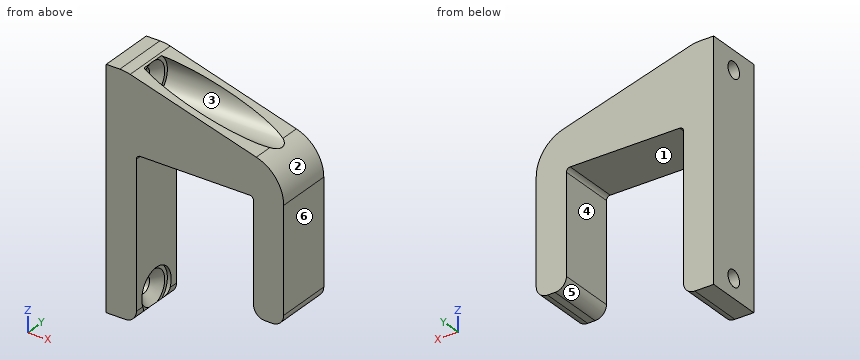
from build123d import *

# Parameters (mm, degrees)
BOSS_EXTRU_1_DEPTH                           = 7.5
CONG_1_R                                     = 1
CONG_2_R                                     = 10
CONG_3_R                                     = 3
CHAMBRAGE_POUR_VIS_T_TE_CYLINDRIQUE_AT_COUNT = 2
CHAMBRAGE_POUR_VIS_T_TE_CYLINDRIQUE_AT_PITCH = 52


with BuildPart() as part:
    # Esquisse1 → Boss.-Extru.1 (new, symmetric)
    with BuildSketch(Plane(origin=(0, 0, 0), x_dir=(1, 0, 0), z_dir=(0, 1, 0))):
        Polygon((0, 0), (0, 42), (-8, 42), (-8, -20), (-3, -20), (39, -8), (39, 30), (31, 30), (31, 0), align=None)
    extrude(amount=BOSS_EXTRU_1_DEPTH, both=True)

    # Congé1
    cong_1_edges = [part.edges().sort_by_distance(p)[0] for p in [
        (31, 0, 0),
        (0, 0, 0),
    ]]
    fillet(cong_1_edges, radius=CONG_1_R)

    # Congé2
    cong_2_edges = [part.edges().sort_by_distance(p)[0] for p in [
        (39, 0, 8),
        (-3, 0, 20),
    ]]
    fillet(cong_2_edges, radius=CONG_2_R)

    # Congé3
    cong_3_edges = [part.edges().sort_by_distance(p)[0] for p in [
        (31, 0, -30),
        (39, 0, -30),
        (0, 0, -42),
    ]]
    fillet(cong_3_edges, radius=CONG_3_R)

    # Esquisse2 → Chambrage pour vis à tête cylindrique à 6 pans creux (ou vis CHC) M41 (revolve, cut)
    with BuildSketch(Plane(origin=(0, 0, -37), x_dir=(0, 0, -1), z_dir=(0, 1, 0))):
        Polygon((0, 0), (0, 8), (2.15, 8), (2.15, 3.35), (4.5, 1), (5.5, 1), (5.5, 0), (5.5, -39), (0, -39), align=None)
    chambrage_pour_vis_t_te_cylindrique = revolve(axis=Axis((6.35, 0, -37), (-1, 0, 0)), mode=Mode.SUBTRACT)

    # Chambrage pour vis à tête cylindrique à 6 pans creux (ou vis CHC) M41 at: Chambrage pour vis à tête cylindrique à 6 pans creux (ou vis CHC) M41 ×2
    with Locations(*[(0, 0, i * CHAMBRAGE_POUR_VIS_T_TE_CYLINDRIQUE_AT_PITCH) for i in range(1, CHAMBRAGE_POUR_VIS_T_TE_CYLINDRIQUE_AT_COUNT)]):
        add(chambrage_pour_vis_t_te_cylindrique, mode=Mode.SUBTRACT)


solid = part.part
Design review of the part built by this model. Coordinates are the model's own, in mm. Face numbers are marked on the shaded views. A direction names the side the tool comes from. Coordinates: 2 decimals unless noted, no trailing zeros. Write each loop counter-clockwise with the first axis right and the second up, starting at its lowest first coordinate (ties: lowest second). Pieces come first, ordered by that corner, then holes. Notation, with made-up numbers: (-18.5, 81.25) - (-7.5, 81.25) arc R23 cw to (-7.5, 104.25) - close; hole circle Ø1 at (-39, 40). An arc over 180 degrees is marked (long way). Use one line per item in the form item = value.
Q1. Consider section A-A (z = -18). Write out the cut boundary in (x, y), plus the area to 3 significant figures.
Taken from the geometry:
outline = (-8, -7.5) - (0, -7.5) - (0, 7.5) - (-8, 7.5) - close; (31, -7.5) - (39, -7.5) - (39, 7.5) - (31, 7.5) - close
area = 240 mm^2
Q2. Consider section D-D (x = 21). Write out the cut boundary in (y, z).
Taken from the geometry:
outline = (-7.5, 0) - (7.5, 0) - (7.5, 13.14) - (5.18, 13.14) arc R5.5 cw to (-5.18, 13.14) - (-7.5, 13.14) - close
Q3. Insertion check: pin 1 Ø12 at (x, z) = (22, -13.5) entering from -Y; pin 2 Ø2 at (x, y) = (23, -0.5) entering from -Z; pin 3 Ø2 at (x, y) = (17.5, 5.5) entering from +Z; pin 4 Ø1 at (x, y) = (0.5, -1.5) entering from +Z. Each pin has a flat end and moves straight along its axis. Give the tip position at first contact, or say it passes through.
Taken from the geometry:
pin_1 = through
pin_2 = 0
pin_3 = 14.43
pin_4 = 9.88
Q4. Machinability: for the marked faces 5 and 6, which of the approach directions +Z, -Z, +X, -X, +Y, -Y give a long, thin tool a straight path to every point of the face, cutting with its end or side? Answer none if there is none.
Taken from the geometry:
face_5 = -Z, +Y, -Y
face_6 = +Z, -Z, +X, +Y, -Y
Q5. Consider section B-B (z = -37). Write out the cut boundary in (x, y).
Taken from the geometry:
outline = (-8, -7.5) - (0, -7.5) - (0, -5.5) - (-1, -5.5) - (-1, -4.5) - (-3.35, -2.15) - (-8, -2.15) - close; (-8, 2.15) - (-3.35, 2.15) - (-1, 4.5) - (-1, 5.5) - (0, 5.5) - (0, 7.5) - (-8, 7.5) - close
Q6. The part is to be moulded in two halves that separate along Z. For the marked faces 1, 2, 3 and 4, say which applies: +Z half, -Z half, draft (parallel to the pull), parting line (faces both ways), or undercut.
Taken from the geometry:
face_1 = -Z half
face_2 = +Z half
face_3 = undercut
face_4 = draft
Q7. Consider section C-C (y = 0). Count the separate pieces of the cut face and the enclosed holes in it, plus the area to 3 significant figures.
Taken from the geometry:
separate_pieces = 3
enclosed_holes = 0
area = 995 mm^2
Q8. For probe 1 along Z at (x, y) = (-4.25, 0); probe 2 along X at (y, z) = (-5.5, -25.5); probe 3 along Y at (x, z) = (8.5, 15), list the stretches that pass through material, from the lowest coordinate up.
Taken from the geometry:
probe_1 = -42 to -39.15, -34.85 to 12.85, 17.15 to 20
probe_2 = -8 to 0, 31 to 39
probe_3 = -7.5 to -5.5, 5.5 to 7.5
